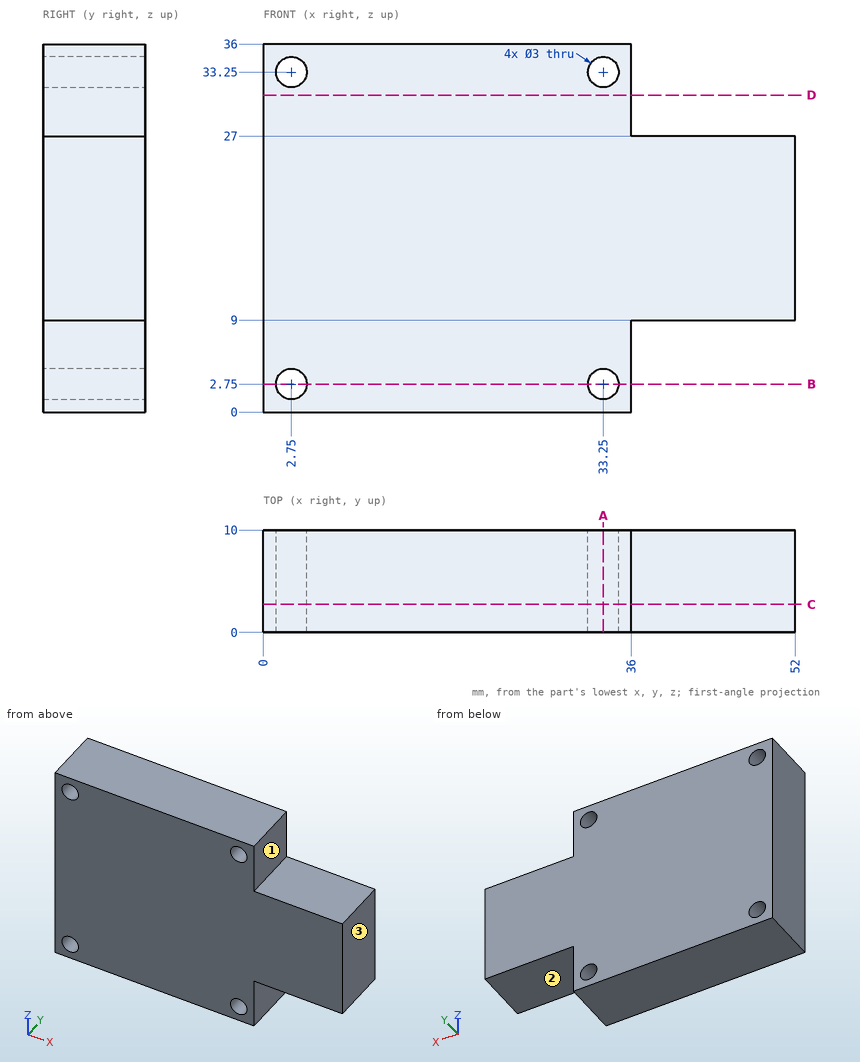
Design review of the part shown in the three views and the two pictorial views. Dimensions are in mm from the part's minimum x, y and z. A direction names the side the tool comes from. Give positions to 0.01 mm unless a question says otherwise; leave off trailing zeros. Order: outer loops, then holes, each group sorted by start corner. A loop starts at its lowest first (then second) coordinate and runs counter-clockwise, first axis right, second up. Notation, with made-up numbers: M -14,-3.75 L 29,-3.75 A34 ccw 29,29.25 Z; hole C -19.75,38 d4. An arc over 180 degrees is marked long. Answer in a Markdown table with one row per item. Add a question column.
(1) Wall thickness on probe 1 along X at (y, z) = (4.25, 33.25); probe 2 along X at (y, z) = (3, 29); probe 3 along Z at (x, y) = (46.5, 7): over which ranges is each line inside the solid? List them lowest first. Write a range as [from, to].
(2) For pin 1 (2.5 mm diameter, centred on x = 33.25, z = 33.25, fed in from -Y), flat-tipped, find the tip position at first contact; note if it passes through.
(3) Consider section C-C on y = 2.75. State the section outline as (x, z) points.
(4) Consider section B-B on z = 2.75. State the section outline as (x, y) points, and give its area (3 significant figures).
(5) Consider section D-D on z = 31. State the section outline as (x, y) points.
(6) Consider section A-A on x = 33.25. State the section outline as (y, z) points.
(7) For the marked faces 1, 2 and 3, list the 3-axis set-ups (+Z, -Z, +X, -X, +Y, -Y) from which the entire face can be reached by the end or side of a thin tool; tool diameter is ignored.
Evaluation:
| question | item | result |
|---|---|---|
| 1 | probe 1 | x = [0, 1.25], [4.25, 31.75], [34.75, 36] |
| 1 | probe 2 | x = [0, 36] |
| 1 | probe 3 | z = [9, 27] |
| 2 | pin 1 | passes through |
| 3 | outline | M 0,0 L 36,0 L 36,9 L 52,9 L 52,27 L 36,27 L 36,36 L 0,36 Z; hole C 2.75,2.75 d3; hole C 2.75,33.25 d3; hole C 33.25,2.75 d3; hole C 33.25,33.25 d3 |
| 4 | outline | M 0,0 L 1.25,0 L 1.25,10 L 0,10 Z; M 4.25,0 L 31.75,0 L 31.75,10 L 4.25,10 Z; M 34.75,0 L 36,0 L 36,10 L 34.75,10 Z |
| 4 | area | 300 mm^2 |
| 5 | outline | M 0,0 L 36,0 L 36,10 L 0,10 Z |
| 6 | outline | M 0,0 L 10,0 L 10,1.25 L 0,1.25 Z; M 0,4.25 L 10,4.25 L 10,31.75 L 0,31.75 Z; M 0,34.75 L 10,34.75 L 10,36 L 0,36 Z |
| 7 | face 1 | +Z, +X, +Y, -Y |
| 7 | face 2 | -Z, +X, +Y, -Y |
| 7 | face 3 | +Z, -Z, +X, +Y, -Y |
